```python
from build123d import *
from OCP.BRepFilletAPI import BRepFilletAPI_MakeChamfer

# Parameters (mm, degrees)
SKETCH2_W                    = 60.7822
SKETCH2_H                    = 279.4
BASE_FLANGE1_DEPTH           = 3.2639
EDGE_FLANGE1_DEPTH           = 101.6
EDGE_FLANGE1_BEND_DEPTH      = 101.6
CHAMFER1_SIZE                = 34.925
CHAMFER1_SIZE2               = 29.305554619
F_10_0_1935_DIAMETER_HOLE1_D = 4.9149
F_1_4_START                  = -3.2639
F_1_4_CLEARANCE_SLOT1_DEPTH  = 3.2639
SKETCH17_W                   = 7.7978
SKETCH17_H                   = 38.1
BOSS_EXTRUDE1_DEPTH          = 3.2639
FILLET1_R                    = 3.175
FILLET2_R                    = 6.35


# Read off the part's stored shape, not the designer's step: 1/4 Clearance Slot1
# Sheet-metal steps are written as plain solids
with BuildPart() as part:
    # Sketch2 → Base-Flange1 (new body)
    with BuildSketch(Plane.XY):
        with Locations((0, 139.7)):
            Rectangle(SKETCH2_W, SKETCH2_H)
    extrude(amount=-BASE_FLANGE1_DEPTH)

    # Edge-Flange1 section (across the edge) → Edge-Flange1 (add)
    with BuildSketch(Plane(origin=(31.6611, 114.3, -3.2639), x_dir=(-1, 0, 0), z_dir=(0, -1, 0))):
        with BuildLine():
            Line((-3.2639, 1.27), (-3.2639, 34.8361))
            Line((-3.2639, 34.8361), (0, 34.8361))
            Line((0, 34.8361), (0, 1.27))
            ThreePointArc((0, 1.27), (0.371974388, 0.371974388), (1.27, 0))
            Line((1.27, 0), (1.27, -3.2639))
            ThreePointArc((1.27, -3.2639), (-1.935951435, -1.935951435), (-3.2639, 1.27))
        make_face()
    extrude(amount=EDGE_FLANGE1_DEPTH)

    # Edge-Flange1 section 2 (across the edge) → Edge-Flange1 bend (add)
    with BuildSketch(Plane(origin=(-31.6611, 12.7, -3.2639), x_dir=(1, 0, 0), z_dir=(0, 1, 0))):
        with BuildLine():
            Line((-3.2639, 1.27), (-3.2639, 34.8361))
            Line((-3.2639, 34.8361), (0, 34.8361))
            Line((0, 34.8361), (0, 1.27))
            ThreePointArc((0, 1.27), (0.371974388, 0.371974388), (1.27, 0))
            Line((1.27, 0), (1.27, -3.2639))
            ThreePointArc((1.27, -3.2639), (-1.935951435, -1.935951435), (-3.2639, 1.27))
        make_face()
    extrude(amount=EDGE_FLANGE1_BEND_DEPTH)

    # Chamfer1: one chamfer whose edges measure the first distance from different faces: ONE call of the kernel's chamfer builder (chamfer() names one face for all edges)
    chamfer1_edges_1 = [part.edges().sort_by_distance(p)[0] for p in [
        (33.29305, 12.7, -38.1),
    ]]
    chamfer1_side_1 = [part.faces().sort_by_distance(p)[0] for p in [
        (33.29305, 63.5, -38.1),
    ]]
    chamfer1_edges_2 = [part.edges().sort_by_distance(p)[0] for p in [
        (-33.29305, 12.7, -38.1),
    ]]
    chamfer1_side_2 = [part.faces().sort_by_distance(p)[0] for p in [
        (-33.29305, 63.5, -38.1),
    ]]
    chamfer1 = BRepFilletAPI_MakeChamfer(part.part.solid().wrapped)
    for e in chamfer1_edges_1:
        chamfer1.Add(CHAMFER1_SIZE, CHAMFER1_SIZE2, e.wrapped, chamfer1_side_1[0].wrapped)  # the first distance lies on this face
    for e in chamfer1_edges_2:
        chamfer1.Add(CHAMFER1_SIZE, CHAMFER1_SIZE2, e.wrapped, chamfer1_side_2[0].wrapped)  # the first distance lies on this face
    add(Compound.cast(chamfer1.Shape()), mode=Mode.REPLACE)

    # #10 (0.1935) Diameter Hole1 (through all)
    with Locations(Plane(origin=(34.925, 0, 0), x_dir=(0, 0, -1), z_dir=(1, 0, 0))):
        with Locations((22.225, 104.775), (22.225, 77.7875), (22.225, 50.8), (12.7, 28.575)):
            Hole(F_10_0_1935_DIAMETER_HOLE1_D / 2)

    # 1/4 Clearance Slot1 outline → 1/4 Clearance Slot1 (cut)
    with BuildSketch(Plane.XY.offset(F_1_4_START)):
        with BuildLine():
            ThreePointArc((-17.2593, 253.7968), (-20.6375, 257.175), (-24.0157, 253.7968))
            Line((-24.0157, 253.7968), (-24.0157, 222.4532))
            ThreePointArc((-24.0157, 222.4532), (-20.6375, 219.075), (-17.2593, 222.4532))
            Line((-17.2593, 222.4532), (-17.2593, 253.7968))
        make_face()
        with BuildLine():
            ThreePointArc((24.0157, 253.7968), (20.6375, 257.175), (17.2593, 253.7968))
            Line((17.2593, 253.7968), (17.2593, 222.4532))
            ThreePointArc((17.2593, 222.4532), (20.6375, 219.075), (24.0157, 222.4532))
            Line((24.0157, 222.4532), (24.0157, 253.7968))
        make_face()
    extrude(amount=F_1_4_CLEARANCE_SLOT1_DEPTH, mode=Mode.SUBTRACT)

    # Sketch17 → Boss-Extrude1 (add)
    with BuildSketch(Plane(origin=(0, 0, -3.2639), x_dir=(-1, 0, 0), z_dir=(0, 0, -1))):
        with Locations((-34.29, 238.125)):
            Rectangle(SKETCH17_W, SKETCH17_H)
        with Locations((34.29, 238.125)):
            Rectangle(SKETCH17_W, SKETCH17_H)
    extrude(amount=-BOSS_EXTRUDE1_DEPTH)

    # Fillet1
    fillet1_edges = [part.edges().sort_by_distance(p)[0] for p in [
        (30.3911, 219.075, -1.63195),
        (30.3911, 257.175, -1.63195),
        (38.1889, 257.175, -1.63195),
        (38.1889, 219.075, -1.63195),
        (-38.1889, 257.175, -1.63195),
        (-38.1889, 219.075, -1.63195),
        (-30.3911, 219.075, -1.63195),
        (-30.3911, 257.175, -1.63195),
        (33.29305, 114.3, -38.1),
        (-33.29305, 114.3, -38.1),
        (33.29305, 47.625, -38.1),
        (33.29305, 12.7, -8.794445381),
        (-33.29305, 12.7, -8.794445381),
        (-33.29305, 47.625, -38.1),
    ]]
    fillet(fillet1_edges, radius=FILLET1_R)

    # Fillet2
    fillet2_edges = [part.edges().sort_by_distance(p)[0] for p in [
        (-30.3911, 279.4, -1.63195),
        (30.3911, 279.4, -1.63195),
        (30.3911, 0, -1.63195),
        (-30.3911, 0, -1.63195),
    ]]
    fillet(fillet2_edges, radius=FILLET2_R)


solid = part.part
```
Geometry check sheet. Reference: the model listing, model coordinates, mm. A direction names the side the tool comes from. Round coordinates to 2 decimals unless told otherwise and drop trailing zeros. Loops run counter-clockwise (first coordinate to the right, second up) from the corner with the lowest first, then second, coordinate; pieces in that order, holes last. Notation, with made-up numbers: (72, -17.75) - (105, -17.75) arc R18 ccw to (105, 1.25) - close; hole circle Ø6 at (-40, 24.5). An arc over 180 degrees is marked (long way). Write each question's results on one line, items separated by ' | '. Start each with the question number.
Q1. Release check for a two-part mould opening along Z. For faces 1 (the flat face through (-33, 12.7, -4)), 2 (the cylindrical face through (33.27, 107.212, -22.545)), 3 (the flat face through (33.32, 30.06, -23.36)) record: +Z half, -Z half, draft (parallel to the pull), parting line (faces both ways), or undercut.
Q2. Access from +Z, -Z, +X, -X, +Y, -Y to the whole of each face (thin tool, end or side, straight path). Record for faces 4 (the flat face through (33, 114.3, -18)), 5 (the flat face through (33, 12.7, -4)), 6 (the flat face through (-33, 114.3, -18)).
Q3. Cross-section at C-C on x = 12. Enter the section's corners in (y, z), and give its area (3 significant figures).
Q4. Cross-section at A-A on z = -12.7. Enter the section's corners in (x, y) (3 decimals).
Q5. Thickness scan on line 1 (X direction, y = 36.5, z = -6) (3 decimals); line 2 (Z direction, x = 26, y = 228.5); line 3 (Y direction, x = 33, z = -12). Record the ranges inside material, lowest first. Write a range as [from, to].
Q6. Cross-section at B-B on y = 118. Enter the section's corners in (x, z).
Q7. Gauge pin test, flat ends, axial feed: P1, Ø1.4, axis at x = -33, z = -5.5, coming from the -Y side; P2, Ø3.5, axis at y = 175, z = -2, coming from the +X side; P3, Ø5.5, axis at y = 77.79, z = -22.22, coming from the +X side (3 decimals). Record the tip position at first contact, or that the pin passes through.
Answers below:
1) face 1: draft | face 2: undercut | face 3: -Z half
2) face 4: +Z, -Z, +X | face 5: +Z, -Z, +X, -Y | face 6: +Z, -Z, -X
3) outline: (0, -3.26) - (279.4, -3.26) - (279.4, 0) - (0, 0) - close | area: 912 mm²
4) outline: (-34.925, 17.354) - (-31.661, 17.354) - (-31.661, 26.118) - (-34.925, 26.118) - close; (-34.925, 31.032) - (-31.661, 31.032) - (-31.661, 114.3) - (-34.925, 114.3) - close; (31.661, 17.354) - (34.925, 17.354) - (34.925, 26.118) - (31.661, 26.118) - close; (31.661, 31.032) - (34.925, 31.032) - (34.925, 114.3) - (31.661, 114.3) - close
5) line 1: x = [-34.925, -31.661], [31.661, 34.925] | line 2: z = [-3.26, 0] | line 3: y = [16.52, 26.22], [30.93, 114.3]
6) outline: (-30.39, -3.26) - (30.39, -3.26) - (30.39, 0) - (-30.39, 0) - close
7) P1: stops at y = 12.7 | P2: stops at x = 30.39 | P3: stops at x = 34.925
